```python
from build123d import *

# Parameters (mm, degrees)
SKETCH1_W           = 3.05
SKETCH1_H           = 6.05
SKETCH1_R           = 3
BOSS_EXTRUDE1_DEPTH = 3
FILLET1_R           = 15
FILLET2_R           = 0.1


with BuildPart() as part:
    # Sketch1 → Boss-Extrude1 (new body)
    with BuildSketch(Plane.XY):
        with BuildLine():
            Line((-32.74355653, 42.5), (-58.5, 42.5))
            ThreePointArc((-58.5, 42.5), (-69.106601718, 38.106601718), (-73.5, 27.5))
            Line((-73.5, 27.5), (-73.5, -42.5))
            Line((-73.5, -42.5), (73.5, -42.5))
            Line((73.5, -42.5), (73.5, -27.5))
            ThreePointArc((73.5, -27.5), (71.490381057, -20), (66, -14.509618943))
            Line((66, -14.509618943), (-32.74355653, 42.5))
        make_face()
        with BuildLine():
            ThreePointArc((-48.5, -27.5), (-51.500000015, -30.5), (-54.5, -27.499999969))
            ThreePointArc((-54.5, -27.499999969), (-50.649618339, 1.746552215), (-39.36087052, 29.000000186))
            ThreePointArc((-39.36087052, 29.000000186), (-35.262794319, 30.098076155), (-34.16471821, 25.999999992))
            ThreePointArc((-34.16471821, 25.999999992), (-44.854063414, 0.193637821), (-48.5, -27.5))
        make_face(mode=Mode.SUBTRACT)
        with Locations((-70, -37.5)):
            Rectangle(SKETCH1_W, SKETCH1_H, mode=Mode.SUBTRACT)
        with Locations((-70, 2.5)):
            Rectangle(SKETCH1_W, SKETCH1_H, mode=Mode.SUBTRACT)
        with Locations((58.5, -27.5)):
            Circle(SKETCH1_R, mode=Mode.SUBTRACT)
    extrude(amount=BOSS_EXTRUDE1_DEPTH)

    # Fillet1
    fillet1_edges = [part.edges().sort_by_distance(p)[0] for p in [
        (-32.74355653, 42.5, 1.5),
    ]]
    fillet(fillet1_edges, radius=FILLET1_R)

    # Fillet2
    fillet2_edges = [part.edges().sort_by_distance(p)[0] for p in [
        (-68.475, -0.525, 1.5),
        (-68.475, 5.525, 1.5),
        (-71.525, 5.525, 1.5),
        (-71.525, -0.525, 1.5),
        (-68.475, -34.475, 1.5),
        (-71.525, -34.475, 1.5),
        (-71.525, -40.525, 1.5),
        (-68.475, -40.525, 1.5),
    ]]
    fillet(fillet2_edges, radius=FILLET2_R)


solid = part.part
```
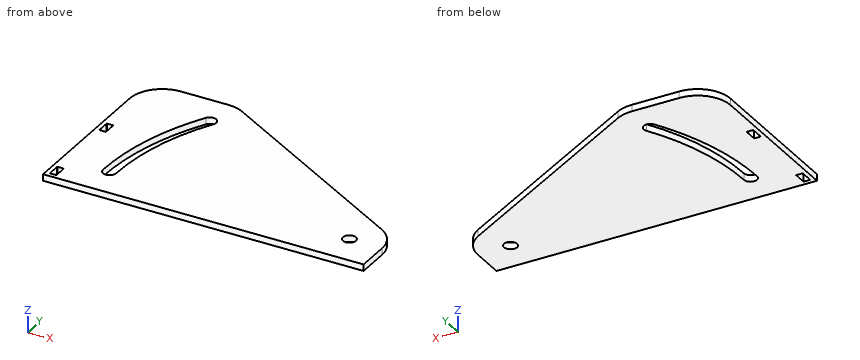
Verification items for the finished model (mm, model axes). Round coordinates to 2 decimals unless told otherwise and drop trailing zeros. Write each loop counter-clockwise with the first axis right and the second up, starting at its lowest first coordinate (ties: lowest second). Pieces come first, ordered by that corner, then holes.
1. Gauge pin test, flat end, axial feed: P1, Ø1.4, axis at x = -70.5, z = 1.5, coming from the +Y side. Record the tip position at first contact, or that the pin passes through.
2. Section check D-D on x = -17.5. Enter the section's corners in (y, z).
3. Section check B-B on x = 58.5. Enter the section's corners in (y, z), plus the area to 3 significant figures.
4. Section check C-C on y = 23. Enter the section's corners in (x, z), plus the area to 3 significant figures.
5. Scan lines: L1, parallel to X at y = -36, z = 2.25 (3 decimals); L2, parallel to X at y = -12, z = 1.8; L3, parallel to X at y = 0, z = 1.15 (3 decimals). Record each from-to range of solid material in increasing order.
6. Section check A-A on z = 2.3. State how many separate pieces and enclosed holes the cut face has, plus the area to 3 significant figures.
Answer:
1. P1: stops at y = 37.36
2. outline: (-42.5, 0) - (33.7, 0) - (33.7, 3) - (-42.5, 3) - close
3. outline: (-42.5, 0) - (-30.5, 0) - (-30.5, 3) - (-42.5, 3) - close; (-24.5, 0) - (-10.18, 0) - (-10.18, 3) - (-24.5, 3) - close
3. area: 79.0 mm2
4. outline: (-73.5, 0) - (-42.59, 0) - (-42.59, 3) - (-73.5, 3) - close; (-35.83, 0) - (1.03, 0) - (1.03, 3) - (-35.83, 3) - close
4. area: 203 mm2
5. L1: x = -73.5 to -71.525, -68.475 to 73.5
5. L2: x = -73.5 to -53.43, -47.37 to 61.65
5. L3: x = -73.5 to -71.525, -68.475 to -51.103, -44.906 to 40.869
6. separate pieces: 1
6. enclosed holes: 4
6. area: 8,740 mm2
